The drawing under review shows one solid part. Ordinate dimensions are in mm from its lowest x, y, z. Round coordinates to 2 decimals unless told otherwise and drop trailing zeros. Order: outer loops, then holes, each group sorted by start corner. A loop starts at its lowest first (then second) coordinate and runs counter-clockwise, first axis right, second up.
1) Consider section A-A (y = 3.5). Give the boundary of the cut face in (x, z), then the cut area to 3 significant figures.
2) Consider section B-B (x = 2.5). Give the boundary of the cut face in (y, z), then the cut area to 3 significant figures.
3) Clearance check with flat-ended pins moving along their axes: P1, Ø0.9, axis at x = 1.5, z = 67, coming from the -Y side; P2, Ø0.9, axis at x = 1.5, z = 112.5, coming from the -Y side. State where each tip first meets the part, or that it passes through.
4) To check wall thickness, follow L1, parallel to Z at x = 1.9, y = 15.5; L2, parallel to Y at x = 1.75, z = 69.5; L3, parallel to Y at x = 1.85, z = 31.5. State the ranges of each line that lie inside material, in increasing order.
5) Consider section C-C (z = 61.5). Give the boundary of the cut face in (x, y).
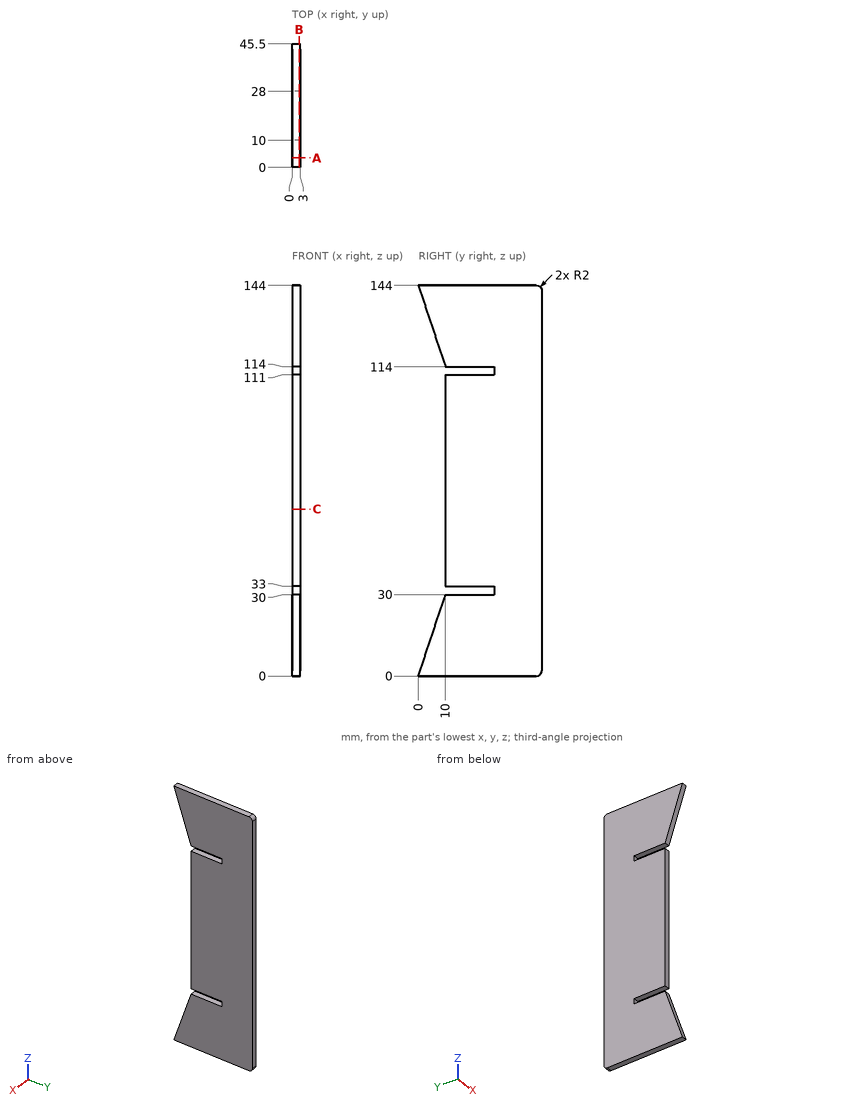
Answer below:
1. outline: (0, 0) - (3, 0) - (3, 10.5) - (0, 10.5) - close; (0, 133.5) - (3, 133.5) - (3, 144) - (0, 144) - close
1. area: 63.0 mm2
2. outline: (0, 0) - (43.5, 0) arc R2 ccw to (45.5, 2) - (45.5, 142) arc R2 ccw to (43.5, 144) - (0, 144) - (10, 114) - (28, 114) - (28, 111) - (10, 111) - (10, 33) - (28, 33) - (28, 30) - (10, 30) - close
2. area: 5,300 mm2
3. P1: stops at y = 10
3. P2: stops at y = 28
4. L1: z = 0 to 30, 33 to 111, 114 to 144
4. L2: y = 10 to 45.5
4. L3: y = 28 to 45.5
5. outline: (0, 10) - (3, 10) - (3, 45.5) - (0, 45.5) - close
